Part model, mm, in its own coordinate system. A direction names the side the tool comes from. Coordinates: 2 decimals unless noted, no trailing zeros. Order: outer loops, then holes, each group sorted by start corner. A loop starts at its lowest first (then second) coordinate and runs counter-clockwise, first axis right, second up.
1) Tool access for faces 1 (the flat face through (-34.5, 1, 42)), 2 (the flat face through (27, 1, -20)), 3 (the flat face through (27, 1, 20)): list every direction of +Z, -Z, +X, -X, +Y, -Y with a clear straight run to the whole face (end or side of a thin tool).
2) Pin check, flat tips, straight feed: pin 1 Ø5 at (x, z) = (-39.75, 18.75) entering from -Y; pin 2 Ø1.5 at (x, y) = (-41, 1.5) entering from +Z; pin 3 Ø1.5 at (x, y) = (-37, 1.5) entering from -Z; pin 4 Ø1.5 at (x, y) = (23, 0.5) entering from -Z. Stop position of each tip, or through.
3) Cut at D-D (y = 0.8). Give the number of separate pieces and of enclosed holes in the cut face, and give its area (3 significant figures).
4) Cut at C-C (z = 42.5). List the corners of the cut face in (x, y), and give its area (3 significant figures).
5) Cut at B-B (x = -28.5). List the corners of the cut face in (y, z).
6) Cut at A-A (z = -13). List the corners of the cut face in (x, y).
7) Mould opens along X. For faces 4 (the cylindrical face through (-3.86, 1.48, -22.35)), 5 (the cylindrical face through (38.522, 1.479, 12.534)), 6 (the flat face through (-12, 1, -47.5)), 7 (the flat face through (9, 1, -34)) say: +X half, -X half, draft (parallel to the pull), parting line (faces both ways), or undercut.
8) Wall check: L1, parallel to Z at x = 14, y = 0.6; L2, parallel to Z at x = -39.75, y = 1.95; L3, parallel to X at y = 0.8, z = 21.5. Give the ranges that are in metal, low to high.
Autodesk Inventor part; units mm, degrees
ref_plane "YZ Plane" through (0, 0, 0) normal (1, 0, 0) x (0, 1, 0)
ref_plane "XZ Plane" through (0, 0, 0) normal (0, 1, 0) x (-1, 0, 0)
ref_plane "XY Plane" through (0, 0, 0) normal (0, 0, 1) x (1, 0, 0)
sketch "Sketch1" plane through (0, 0, 0) normal (0, 1, 0) x (-1, 0, 0)
  line L0 (-45, 0) -> (-45, 6)
  line L1 (-45, 6) -> (-45, -6)
  line L2 (-45, 6) -> (-45, 20)
  line L3 (-45, 20) -> (-45, -6)
  line L4 (-45, -6) -> (-45, -20)
  line L5 (-45, 20) -> (-9, 20)
  line L6 (-45, -20) -> (-9, -20)
  line L7 (-45, -20) -> (-9, -20)
  line L8 (-9, 20) -> (-9, 47.5)
  line L9 (-45, 6) -> (-45, 20)
  circle A0 centre (-14, 13) radius 1.55
  circle A1 centre (-14, -13) radius 1.55
  circle A2 centre (-40, 13) radius 1.55
  circle A3 centre (-40, -13) radius 1.55
  line L10 (-45, 20) -> (-45, -20)
  line L11 (-9, 20) -> (-45, 20)
  line L12 (-45, 20) -> (-45, -20)
  line L13 (-45, -20) -> (-9, -20)
  line L14 (45, 37.5) -> (34.5, 37.5)
  line L15 (45, -37.5) -> (34.5, -37.5)
  line L16 (34.5, -37.5) -> (34.5, -47.5)
  line L17 (34.5, 37.5) -> (34.5, 47.5)
  circle A4 centre (28.5, 42.5) radius 1.55
  circle A5 centre (28.5, -42.5) radius 1.55
  line L18 (34.5, -47.5) -> (-5, -47.5)
  line L19 (45, -37.5) -> (45, 37.5)
  line L20 (34.5, 47.5) -> (-9, 47.5)
  line L21 (-9, -20) -> (-9, -47.5)
  line L22 (-9, -47.5) -> (-5, -47.5)
  circle A6 centre (5, 21.3) radius 1.55
  circle A7 centre (5, -21.3) radius 1.55
  circle A8 centre (39.75, 18.75) radius 1.55
  circle A9 centre (39.75, 0) radius 1.55
  circle A10 centre (39.75, -18.75) radius 1.55
  point P0 (0, 0)
  dimension "d2" = 6
  dimension "d3" = 12
  dimension "d4" = 14
  dimension "d5" = 14
  dimension "d6" = 36
  dimension "d7" = 36
  dimension "d13" = 3.1
  dimension "d14" = 3.1
  dimension "d15" = 3.1
  dimension "d17" = 10.5
  dimension "d19" = 10.5
  dimension "d22" = 3.1
  dimension "d23" = 3.1
  dimension "d27" = 3.1
  dimension "d28" = 3.1
  dimension "d32" = 3.1
  dimension "d33" = 3.1
  dimension "d34" = 3.1
extrude "Extrusion2" add sketch "Sketch1" along normal blind 3
properties part number "basePlate"
Geometry check:
1. face 1: +Z, -X, +Y, -Y
1. face 2: -Z, +X, +Y, -Y
1. face 3: +Z, +X, +Y, -Y
2. pin 1: stops at y = 0
2. pin 2: stops at z = 37.5
2. pin 3: stops at z = -37.5
2. pin 4: stops at z = -20
3. separate pieces: 1
3. enclosed holes: 11
3. area: 6,280 mm2
4. outline: (-34.5, 0) - (-30.05, 0) - (-30.05, 3) - (-34.5, 3) - close; (-26.95, 0) - (9, 0) - (9, 3) - (-26.95, 3) - close
4. area: 121 mm2
5. outline: (0, -47.5) - (3, -47.5) - (3, -44.05) - (0, -44.05) - close; (0, -40.95) - (3, -40.95) - (3, 40.95) - (0, 40.95) - close; (0, 44.05) - (3, 44.05) - (3, 47.5) - (0, 47.5) - close
6. outline: (-45, 0) - (12.45, 0) - (12.45, 3) - (-45, 3) - close; (15.55, 0) - (38.45, 0) - (38.45, 3) - (15.55, 3) - close; (41.55, 0) - (45, 0) - (45, 3) - (41.55, 3) - close
7. face 4: undercut
7. face 5: undercut
7. face 6: draft
7. face 7: +X half
8. L1: z = -20 to -14.55, -11.45 to 11.45, 14.55 to 20
8. L2: z = -37.5 to -20.3, -17.2 to -1.55, 1.55 to 17.2, 20.3 to 37.5
8. L3: x = -45 to -6.54, -3.46 to 9
